Can you work these out from the model? Positions are in its coordinate system, mm. Face numbers are marked on the shaded views. A direction names the side the tool comes from. Coordinates: 2 decimals unless noted, no trailing zeros. Order: outer loops, then holes, each group sorted by start corner. A loop starts at its lowest first (then second) coordinate and runs counter-clockwise, first axis right, second up. Notation, with made-up numbers: (-29, 56.25) -> (-17, 56.25) arc R14 cw to (-17, 61.25) -> close; hole circle Ø4 at (-32.75, -12.75). An arc over 180 degrees is marked (long way). Return JSON: item names as keys, results as strings. Group by question number.
1) For pin 1 (5 mm diameter, centred on x = -12.25, y = 7.5, fed in from +Z); pin 2 (8 mm diameter, centred on x = -17.5, z = 12.5, fed in from +Y); pin 3 (4 mm diameter, centred on x = 13.5, y = -10, fed in from +Z), each with a flat end and sliding along its axis, tell me the tip position at first contact or that it passes through.
2) If we section it at D-D, the plane z = 6.5: Please give me the cut outline in (x, y) (3 decimals).
3) For the marked faces 5 and 6, which set-ups out of +Z, -Z, +X, -X, +Y, -Y let a thin tool reach every point of the face, with its end or its side?
4) If we section it at A-A, the plane z = 23.1: Please give me the cut outline in (x, y), then the cut area to 3 significant figures.
5) If I drill on probe 1 along Y at (x, z) = (-12.25, 2.5) (3 decimals); probe 2 along Z at (x, y) = (21, 0); probe 3 along Y at (x, z) = (5, 1.75) (3 decimals), over which ranges is the centre line in solid material (lowest first)? Write a range as from..to.
6) If we section it at B-B, the plane y = 7.5: Please give me the cut outline in (x, z) (3 decimals).
7) If we section it at C-C, the plane x = 20: Please give me the cut outline in (y, z).
8) Thinking about a two-plate mould opening in Y: for the marked faces 1, 2, 3 and 4, which applies, +Y half, -Y half, draft (parallel to the pull), parting line (faces both ways), or undercut?
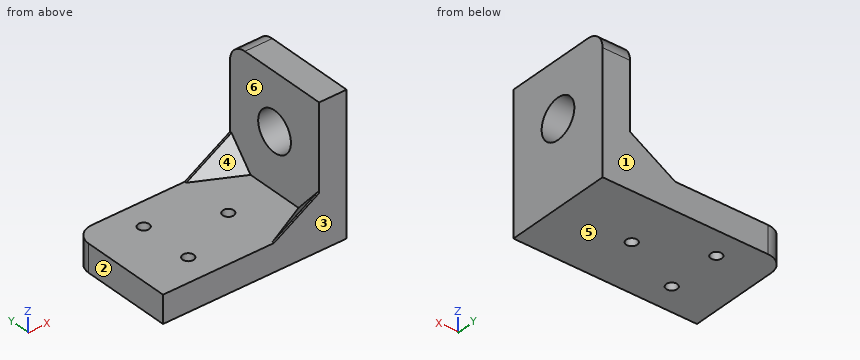
from build123d import *

# Parameters (mm, degrees)
F0_W          = 50.8
F0_H          = 30
F0_R          = 1.525
F1_DEPTH      = 7.6
F2_W          = 7.6
F2_H          = 30
F3_DEPTH      = 31
F4_R          = 5.5
F5_DEPTH      = 7.6
F6_R          = 5
F9_DEPTH      = 7
F10_DEPTH     = 7
F11_T4_DEPTH  = 48.0092585807
F11_T10_DEPTH = 48.0092585807


# Not quite as in the source:
# - a fillet or chamfer that OpenCascade refuses, or shapes differently, is made with other operations: its cross-section is extruded or revolved along the edge and cut away or added


with BuildPart() as f1:
    # F0 (on Top) → F1 (new body)
    with BuildSketch(Plane.XY):
        Rectangle(F0_W, F0_H)
        with Locations((-12.25, -7.5)):
            Circle(F0_R, mode=Mode.SUBTRACT)
        with Locations((-12.25, 7.5)):
            Circle(F0_R, mode=Mode.SUBTRACT)
        with Locations((5, 0)):
            Circle(F0_R, mode=Mode.SUBTRACT)
    extrude(amount=F1_DEPTH)

    # F2 (on face) → F3 (join)
    with BuildSketch(Plane.XY.offset(7.6)):
        with Locations((21.6, 0)):
            Rectangle(F2_W, F2_H)
    extrude(amount=F3_DEPTH)

    # F4 (on face) → F5 (cut)
    with BuildSketch(Plane(origin=(17.8, 0, 0), x_dir=(0, -1, 0), z_dir=(-1, 0, 0))):
        with Locations((0, 23.1)):
            Circle(F4_R)
    extrude(amount=-F5_DEPTH, mode=Mode.SUBTRACT)

    # F6
    f6_edges = [f1.edges().sort_by_distance(p)[0] for p in [
        (21.6, 15, 38.6),
        (-25.4, 15, 3.8),
    ]]
    fillet(f6_edges, radius=F6_R)

    # F7 (on face) → F9 (join)
    with BuildSketch(Plane(origin=(0, 15, 0), x_dir=(-1, 0, 0), z_dir=(0, 1, 0))):
        Polygon((-5.3, 7.6), (-17.8, 15.1), (-17.8, 7.6), align=None)
    extrude(amount=-F9_DEPTH)

    # F8 (on face) → F10 (join)
    with BuildSketch(Plane.XZ.offset(15)):
        Polygon((17.8, 7.6), (17.8, 15.1), (5.3, 7.6), align=None)
    extrude(amount=-F10_DEPTH)

    # F11: chamfer of 6.5 on 2 edges, made by hand


with BuildPart() as f11_tool2:
    # F11_s3 → F11_t4 (new body)
    with BuildSketch(Plane(origin=(-7.0837998008, 0, -4.2502798805), x_dir=(0, 1, 0), z_dir=(0.8574929257, 0, 0.5144957554))):
        Polygon((14.5, 3.7901187316), (8, -2.7098812684), (8, 3.7901187316), align=None)
    extrude(amount=F11_T4_DEPTH)

    split(bisect_by=Plane.YZ.offset(17.8), keep=Keep.BOTTOM)

    split(bisect_by=Plane.XY.offset(7.6), keep=Keep.TOP)


with BuildPart() as f1_1:
    add(f1.part)

    # F11_t1: cut F11_tool2
    add(f11_tool2.part, mode=Mode.SUBTRACT)


with BuildPart() as f11_tool8:
    # F11_s9 → F11_t10 (new body)
    with BuildSketch(Plane(origin=(34.0837998008, 0, 20.4502798805), x_dir=(0, 1, 0), z_dir=(-0.8574929257, 0, -0.5144957554))):
        Polygon((-8, 2.7098812684), (-14.5, -3.7901187316), (-8, -3.7901187316), align=None)
    extrude(amount=F11_T10_DEPTH)

    split(bisect_by=Plane.YZ.offset(17.8), keep=Keep.BOTTOM)

    split(bisect_by=Plane.XY.offset(7.6), keep=Keep.TOP)


with BuildPart() as f1_2:
    add(f1_1.part)

    # F11_t7: cut F11_tool8
    add(f11_tool8.part, mode=Mode.SUBTRACT)


solid = f1_2.part
Result sheet:
{
 "1": {"pin 1": "stops at z = 7.6", "pin 2": "passes through", "pin 3": "stops at z = 9.9"},
 "2": {"outline": "(-25.4, -15) -> (25.4, -15) -> (25.4, 15) -> (-20.4, 15) arc R5 ccw to (-25.4, 10) -> close; hole circle Ø3.05 at (-12.25, -7.5); hole circle Ø3.05 at (-12.25, 7.5); hole circle Ø3.05 at (5, 0)"},
 "3": {"face 5": "-Z, +X, -X, +Y, -Y", "face 6": "+Z, -X"},
 "4": {"outline": "(17.8, -15) -> (25.4, -15) -> (25.4, -5.5) -> (17.8, -5.5) -> close; (17.8, 5.5) -> (25.4, 5.5) -> (25.4, 15) -> (17.8, 15) -> close", "area": "144 mm2"},
 "5": {"probe 1": "y = -15..-9.025, -5.975..5.975, 9.025..15", "probe 2": "z = 0..17.6, 28.6..38.6", "probe 3": "y = -15..-1.525, 1.525..15"},
 "6": {"outline": "(-25.4, 0) -> (-13.775, 0) -> (-13.775, 7.6) -> (-25.4, 7.6) -> close; (-10.725, 0) -> (25.4, 0) -> (25.4, 38.6) -> (17.8, 38.6) -> (17.8, 7.6) -> (-10.725, 7.6) -> close"},
 "7": {"outline": "(-15, 0) -> (15, 0) -> (15, 33.6) arc R5 ccw to (10, 38.6) -> (-15, 38.6) -> close; hole circle Ø11 at (0, 23.1)"},
 "8": {"face 1": "+Y half", "face 2": "draft", "face 3": "-Y half", "face 4": "undercut"}
}
